Read the model definition and answer for the solid it produces. Units are mm, in the model's axes. A direction names the side the tool comes from. Give positions to 0.01 mm unless a question says otherwise; leave off trailing zeros. Write each loop counter-clockwise with the first axis right and the second up, starting at its lowest first coordinate (ties: lowest second). Pieces come first, ordered by that corner, then holes. Notation, with made-up numbers: M 12,-10.75 L 39,-10.75 A20 ccw 39,14.25 Z; hole C -34,64.5 d9. An arc over 180 degrees is marked long. Use a Markdown table: item, result. Add a question column.
Item 1: Consider probe 1 along Z at (x, y) = (-15, 4); probe 2 along Y at (x, z) = (7.5, 11); probe 3 along Y at (x, z) = (33, -8). Determine where each line is inside the solid, lowest interval first. Write a range as [from, to].
Item 2: For faces 4 (the flat face through (-5, 12.5, 0)), 5 (the flat face through (53.85, -4.02, -0.17)), 6 (the flat face through (52.9, -5.15, 13.48)), determine the directions among +Z, -Z, +X, -X, +Y, -Y from which every point of the face is accessible in a straight line to the end or side of a thin tool.
Item 3: The mould has two halves that part along X. Classify faces 1 (the cylindrical face through (24.57, -14.04, 0.17)), 2 (the cylindrical face through (217.892, 6.157, -0.168)), 3 (the flat face through (142.185, 4.902, -0.168)): pulls with the +X half, pulls with the -X half, needs draft (parallel to the pull), parting line crosses it, or undercut.
Item 4: Given P1, Ø10, axis at x = 32.5, z = 7.5, coming from the +Y side; P2, Ø6, axis at x = 66.5, z = 8.5, coming from the +Y side; P3, Ø2, axis at x = 190.5, z = 11, coming from the +Y side, each flat-ended and moving along its own axis, determine where each tip first touches the part or whether it passes through.
Item 5: A cutting plane is placed at A-A on x = -15. Determine the outline of the cut face in (y, z), then the cut area to 3 significant figures.
Autodesk Inventor part; units mm, degrees
ref_plane "YZ Plane" through (0, 0, 0) normal (1, 0, 0) x (0, 1, 0)
ref_plane "XZ Plane" through (0, 0, 0) normal (0, 1, 0) x (-1, 0, 0)
ref_plane "XY Plane" through (0, 0, 0) normal (0, 0, 1) x (1, 0, 0)
sketch "Sketch1" plane through (0, 0, 0) normal (0, 0, 1) x (1, 0, 0)
  line L0 (25, -12.5) -> (-25, -12.5)
  line L1 (-25, -12.5) -> (-25, 12.5)
  line L2 (-25, 12.5) -> (25, 12.5)
  line L3 (25, -12.5) -> (-25, 12.5) construction
  line L4 (-25, -12.5) -> (25, 12.5) construction
  line L5 (25, 12.5) -> (70, 12.5) construction
  line L6 (70, 12.5) -> (70, -17.5) construction
  line L7 (70, -17.5) -> (70, 27.5) construction
  line L8 (70, 27.5) -> (215, 27.5) construction
  line L9 (25, -12.5) -> (64.4199, -45.408)
  line L10 (70, -17.5) -> (41.0213, 6.6916)
  line L11 (70, -17.5) -> (215, 27.5)
  line L12 (215, 27.5) -> (222.41, 3.6234)
  line L13 (222.41, 3.6234) -> (77.41, -41.3766)
  line L14 (41.0213, 6.6916) -> (34.0635, 12.5)
  line L15 (25, 12.5) -> (34.0635, 12.5)
  line L16 (77.41, -41.3766) -> (64.4199, -45.408)
  point P0 (0, 0)
  dimension "d3" = 30
  dimension "d5" = 50
  dimension "d6" = 25
  dimension "d7" = 45
  dimension "d8" = 45
  dimension "d9" = 145
  dimension "d12" = 25
  dimension "d13" = 25
extrude "Extrusion1" add sketch "Sketch1" along normal mid plane 30
fillet "Fillet1" radius 50 1 edges at (34.0635, 12.5, 0)
fillet "Fillet2" radius 25 1 edges at (25, -12.5, 0)
fillet "Fillet3" radius 50 1 edges at (64.4199, -45.408, 0)
fillet "Fillet4" radius 25 1 edges at (70, -17.5, 0)
fillet "Fillet5" radius 12.5 2 edges at (215, 27.5, 0) (222.41, 3.6234, 0)
chamfer "Chamfer1" distance 3 angle 45 18 edges at (32.9782, 9.5062, 15) (53.7689, -3.9502, 15) (143.0261, 5.1633, 15) (212.5886, 22.9184, 15) (150.4361, -18.7133, 15) (65.7768, -38.6215, 15) (37.7476, -23.1418, 15) (-4.5318, -12.5, 15) (-4.5318, 12.5, 15) (32.9782, 9.5062, -15) (-4.5318, 12.5, -15) (53.7689, -3.9502, -15) (143.0261, 5.1633, -15) (212.5886, 22.9184, -15) (150.4361, -18.7133, -15) (65.7768, -38.6215, -15) (37.7476, -23.1418, -15) (-4.5318, -12.5, -15)
sketch "Sketch2" plane through (-25, 12.5, -12) normal (0, 1, 0) x (1, 0, 0)
  line L0 (0, 0) -> (0, -24)
  point P0 (25, -12)
  point P1 (10, -12)
  dimension "d24" = 10
hole "Hole1" at (-15, 12.5, 0) direction (0, -1, 0) diameter 8 end through all
properties part number "Robot_support"
Filled in:
| question | item | result |
|---|---|---|
| 1 | probe 1 | [-15, -4], [4, 15] |
| 1 | probe 2 | [-12.5, 12.5] |
| 1 | probe 3 | [-19.18, 9.5] |
| 2 | face 4 | +Z, -Z, -X, +Y |
| 2 | face 5 | +Z, -Z, +Y |
| 2 | face 6 | +Z, +Y |
| 3 | face 1 | pulls with the -X half |
| 3 | face 2 | pulls with the +X half |
| 3 | face 3 | undercut |
| 4 | P1 | y = 11.14 |
| 4 | P2 | y = -11.48 |
| 4 | P3 | y = 20.21 |
| 5 | outline | M -12.5,-12 L -9.5,-15 L 9.5,-15 L 12.5,-12 L 12.5,-4 L -12.5,-4 Z; M -12.5,4 L 12.5,4 L 12.5,12 L 9.5,15 L -9.5,15 L -12.5,12 Z |
| 5 | area | 532 mm² |
